Can you work these out from the model? Positions are in its coordinate system, mm. Give positions to 0.01 mm unless a question says otherwise; leave off trailing zeros. Order: outer loops, then holes, each group sorted by start corner. A loop starts at its lowest first (then second) coordinate and runs counter-clockwise, first axis right, second up. Notation, with made-up numbers: (26.5, 88) - (75.5, 88) arc R24 ccw to (75.5, 99) - close; hole circle Ø11 at (86.5, 43). An arc over 180 degrees is marked (long way). Use one line per item in the form item = value. Start each with the question number.
1) Suppose I cut it at A-A, the plane y = 10. Write out the boundary of the cut face in (x, z).
2) For pin 1 (8 mm diameter, centred on y = 4.5, z = 5.5, fed in from +X); pin 2 (4 mm diameter, centred on y = 5, z = 4.5, fed in from +X), each with a flat end and sliding along its axis, tell me the tip position at first contact or that it passes through.
3) Suppose I cut it at B-B, the plane z = 12.75. Write out the boundary of the cut face in (x, y), and give its area (3 significant figures).
```python
from build123d import *

# Parameters (mm, degrees)
SKETCH1_W               = 987.806
SKETCH1_H               = 20
BOSS_EXTRUDE1_DEPTH     = 20
CUT_EXTRUDE1_DEPTH      = 20
CUT_EXTRUDE4_DEPTH      = 989.210854846
CUT_EXTRUDE5_DEPTH      = 989.210854846
CUT_EXTRUDE5_DEPTH_BACK = 989.210854846
CUT_EXTRUDE9_DEPTH      = 768.684470274


with BuildPart() as part:
    # Sketch1 → Boss-Extrude1 (new body)
    with BuildSketch(Plane.XY):
        with Locations((493.903, 10)):
            Rectangle(SKETCH1_W, SKETCH1_H)
    extrude(amount=BOSS_EXTRUDE1_DEPTH)

    # Sketch2 → Cut-Extrude1 (cut)
    with BuildSketch(Plane.XY.offset(20)):
        Polygon((0, 20), (0, 0), (54.949548389, 20), align=None)
    extrude(amount=-CUT_EXTRUDE1_DEPTH, mode=Mode.SUBTRACT)

    # Sketch5 → Cut-Extrude4 (cut, through all)
    with BuildSketch(Plane.XY.offset(20)):
        Polygon((987.806, 20), (980.526595315, 0), (987.806, 0), align=None)
    extrude(amount=-CUT_EXTRUDE4_DEPTH, mode=Mode.SUBTRACT)

    # Sketch7 → Cut-Extrude5 (cut, two sides: drawn at the far end of the back side and taken through both)
    with BuildSketch(Plane.XY.offset(20).offset(-CUT_EXTRUDE5_DEPTH_BACK)):
        Polygon((743.328174074, 0), (980.526595315, 0), (987.806, 20), (767.163245926, 20), align=None)
    extrude(amount=CUT_EXTRUDE5_DEPTH + CUT_EXTRUDE5_DEPTH_BACK, mode=Mode.SUBTRACT)

    # Sketch8 → Cut-Extrude9 (cut, through all)
    with BuildSketch(Plane.XY.offset(20)):
        Polygon((743.328174074, 0), (736.048769389, 20), (767.163245926, 20), align=None)
    extrude(amount=-CUT_EXTRUDE9_DEPTH, mode=Mode.SUBTRACT)


solid = part.part
```
Result sheet:
q1.outline = (27.47, 0) - (739.69, 0) - (739.69, 20) - (27.47, 20) - close
q2.pin_1 = 743.15
q2.pin_2 = 742.24
q3.outline = (0, 0) - (743.33, 0) - (736.05, 20) - (54.95, 20) - close
q3.area = 14,200 mm²
